Read the model definition and answer for the solid it produces. Units are mm, in the model's axes. Coordinates: 2 decimals unless noted, no trailing zeros. Order: outer loops, then holes, each group sorted by start corner. A loop starts at its lowest first (then second) coordinate and runs counter-clockwise, first axis right, second up.
```python
from build123d import *

# Parameters (mm, degrees)
SKETCH1_W               = 200
SKETCH1_H               = 200
BOSS_EXTRUDE1_DEPTH     = 4
CUT_EXTRUDE1_DEPTH      = 142.477913471
CUT_EXTRUDE1_DEPTH_BACK = 142.477913471


with BuildPart() as part:
    # Sketch1 → Boss-Extrude1 (new body)
    with BuildSketch(Plane(origin=(0, 0, 0), x_dir=(1, 0, 0), z_dir=(0, 1, 0))):
        Rectangle(SKETCH1_W, SKETCH1_H)
    extrude(amount=BOSS_EXTRUDE1_DEPTH)

    # Sketch2 → Cut-Extrude1 (cut, two sides: drawn at the far end of the back side and taken through both)
    with BuildSketch(Plane(origin=(0, 4, 0), x_dir=(1, 0, 0), z_dir=(0, 1, 0)).offset(-CUT_EXTRUDE1_DEPTH_BACK)):
        Polygon((726.729261237, -609.667248673), (207.718866814, -90.656854249), (-90.656854249, 207.718866814), (-609.667248673, 726.729261237), (428.353540174, 1764.750050084), (1764.750050084, 428.353540174), align=None)
    extrude(amount=CUT_EXTRUDE1_DEPTH + CUT_EXTRUDE1_DEPTH_BACK, mode=Mode.SUBTRACT)


solid = part.part
```
1) A cutting plane is placed at B-B, the plane z = -86. Determine the outline of the cut face in (x, y), and give its area (3 significant figures).
A:
outline: (-100, 0) - (31.06, 0) - (31.06, 4) - (-100, 4) - close
area: 524 mm2
2) A cutting plane is placed at C-C, the plane x = 75.5. Determine the outline of the cut face in (y, z).
A:
outline: (0, -41.56) - (4, -41.56) - (4, 100) - (0, 100) - close
3) Straight lines are drawn through the part: line 1 (Z direction, x = 78, y = 0.85); line 2 (Z direction, x = 27.5, y = 0.2); line 3 (X direction, y = 2.05, z = -42.5). For each, find the intervals that lie inside material, in ascending order.
A:
line 1: z = -39.06 to 100
line 2: z = -89.56 to 100
line 3: x = -100 to 74.56
4) A cutting plane is placed at A-A, the plane y = 0.65. Determine the outline of the cut face in (x, z), and give its area (3 significant figures).
A:
outline: (-100, -100) - (17.06, -100) - (100, -17.06) - (100, 100) - (-100, 100) - close
area: 36,600 mm2
5) A flat-ended cylindrical pin translates along its axis: pin 1 Ø2 at (y, z) = (1, -30.5) entering from +X. Find the tip coordinate at first contact, or state that the pin passes through.
A:
pin 1: stops at x = 87.56
